from build123d import *

# Parameters (mm, degrees)
BOSS_EXTRUDE1_DEPTH            = 9.6
SKETCH2_W                      = 21
SKETCH2_H                      = 15
BOSS_EXTRUDE2_DEPTH            = 2
SKETCH3_W                      = 18.8
SKETCH3_H                      = 13
BOSS_EXTRUDE3_DEPTH            = 13.5
SKETCH4_W                      = 1
SKETCH4_H                      = 4.8
BOSS_EXTRUDE4_DEPTH            = 8
SKETCH5_W                      = 1
SKETCH5_H                      = 4.8
BOSS_EXTRUDE5_DEPTH            = 8
SKETCH6_W                      = 1
SKETCH6_H                      = 4.8
BOSS_EXTRUDE6_DEPTH            = 8
F_1_6_1_6_DIAMETER_HOLE1_D     = 1.6
F_1_6_1_6_DIAMETER_HOLE1_DEPTH = 1
F_1_6_1_6_DIAMETER_HOLE2_D     = 1.6
F_1_6_1_6_DIAMETER_HOLE2_DEPTH = 1
F_1_6_1_6_DIAMETER_HOLE3_D     = 1.6
F_1_6_1_6_DIAMETER_HOLE3_DEPTH = 11
CHAMFER1_SIZE                  = 0.25
CHAMFER2_SIZE                  = 0.5


with BuildPart() as part:
    # Sketch1 → Boss-Extrude1 (new body)
    with BuildSketch(Plane(origin=(0, 0, -4.8), x_dir=(-1, 0, 0), z_dir=(0, 0, -1))):
        with BuildLine():
            Line((-7.639445546, 15.5), (6.803913489, 15.5))
            ThreePointArc((6.803913489, 15.5), (1.329165769, 16.958613053), (-3.894073755, 19.15364916))
            ThreePointArc((-3.894073755, 19.15364916), (-6.290531384, 17.863745283), (-7.639445546, 15.5))
        make_face()
    extrude(amount=-BOSS_EXTRUDE1_DEPTH)

    # Sketch2 → Boss-Extrude2 (add)
    with BuildSketch(Plane(origin=(0, 15.5, 0), x_dir=(1, 0, 0), z_dir=(0, 1, 0))):
        Rectangle(SKETCH2_W, SKETCH2_H)
    extrude(amount=-BOSS_EXTRUDE2_DEPTH)

    # Sketch3 → Boss-Extrude3 (add)
    with BuildSketch(Plane.XZ.offset(-13.5)):
        Rectangle(SKETCH3_W, SKETCH3_H)
    extrude(amount=BOSS_EXTRUDE3_DEPTH)

    # Sketch4 → Boss-Extrude4 (add)
    with BuildSketch(Plane.XZ):
        Rectangle(SKETCH4_W, SKETCH4_H)
    extrude(amount=BOSS_EXTRUDE4_DEPTH)

    # Sketch5 → Boss-Extrude5 (add)
    with BuildSketch(Plane.XZ):
        with Locations((7.1, 0)):
            Rectangle(SKETCH5_W, SKETCH5_H)
    extrude(amount=BOSS_EXTRUDE5_DEPTH)

    # Sketch6 → Boss-Extrude6 (add)
    with BuildSketch(Plane.XZ):
        with Locations((-7.1, 0)):
            Rectangle(SKETCH6_W, SKETCH6_H)
    extrude(amount=BOSS_EXTRUDE6_DEPTH)

    # Ø1.6 (1.6) Diameter Hole1
    with Locations(Plane.ZY.offset(7.6)):
        with Locations((0, -4.5)):
            Hole(F_1_6_1_6_DIAMETER_HOLE1_D / 2, depth=F_1_6_1_6_DIAMETER_HOLE1_DEPTH)

    # Ø1.6 (1.6) Diameter Hole2
    with Locations(Plane(origin=(7.6, 0, 0), x_dir=(0, 0, -1), z_dir=(1, 0, 0))):
        with Locations((0, -4.5)):
            Hole(F_1_6_1_6_DIAMETER_HOLE2_D / 2, depth=F_1_6_1_6_DIAMETER_HOLE2_DEPTH)

    # Ø1.6 (1.6) Diameter Hole3
    with Locations(Plane.ZY.offset(0.5)):
        with Locations((0, -4.5)):
            Hole(F_1_6_1_6_DIAMETER_HOLE3_D / 2, depth=F_1_6_1_6_DIAMETER_HOLE3_DEPTH)

    # Chamfer1
    chamfer1_edges = [part.edges().sort_by_distance(p)[0] for p in [
        (-0.5, -8, 0),
        (0.5, -8, 0),
        (6.6, -8, 0),
        (7.6, -8, 0),
    ]]
    chamfer(chamfer1_edges, length=CHAMFER1_SIZE)

    # Chamfer2
    chamfer2_edges = [part.edges().sort_by_distance(p)[0] for p in [
        (7.1, -8, 2.4),
        (-7.1, -8, -2.4),
        (7.1, -8, -2.4),
        (0, -8, -2.4),
        (-7.1, -8, 2.4),
        (0, -8, 2.4),
    ]]
    chamfer(chamfer2_edges, length=CHAMFER2_SIZE)


solid = part.part
Input: part model. Units: mm. Frame: model coordinates. A direction names the side the tool comes from. Coordinates: 2 decimals unless noted, no trailing zeros. Loops run counter-clockwise (first coordinate to the right, second up) from the corner with the lowest first, then second, coordinate; pieces in that order, holes last. Notation, with made-up numbers: (32.5, -20) - (73.5, -20) arc R32 cw to (73.5, 12) - close; hole circle Ø5 at (62.25, -16.5). An arc over 180 degrees is marked (long way). Answer in a Markdown table with one row per item. Add a question column.
Item 1: Mould query, pull axis Z, two halves, no side actions, for faces 1 (the cylindrical face through (-1.404, 16.933, -0.067)), 2 (the flat face through (0, 7, 6.5)), 3 (the cylindrical face through (-7.09, -5.28, 0.17)). Classes: released by +Z, released by -Z, zero draft, split by the parting line, or undercut.
Item 2: Section query A-A on y = -4.5. Return the cut outline in (x, z).
Item 3: Section query B-B on z = -3. Return the cut outline in (x, y).
Item 4: Contact query for flat-ended pins moving along their axis: P1, Ø4, axis at x = 2, y = -2.5, coming from the +Z side; P2, Ø1.4, axis at y = -3.5, z = -1, coming from the -X side; P3, Ø4, axis at x = 2, z = -5.5, coming from the +Y side; P4, Ø1.4, axis at y = -4.5, z = 0, coming from the +X side. Output: stop coordinate, or through.
Item 5: Section query D-D on z = 0. State how many separate pieces and enclosed holes the cut face has, then the cut area to 3 significant figures.
Item 6: Section query C-C on x = -5. Return the cut outline in (y, z), then the cut area to 3 significant figures.
Item 7: Line query: line 1 along X through (y, z) = (-6.75, 0); line 2 along Y through (x, z) = (-7.25, 0); line 3 along Z through (x, y) = (7, -4.5). Output: solid intervals per line, ascending. Write a range as [from, to].
Item 8: Access query for faces 4 (the flat face through (-7.6, -3, 0)), 5 (the flat face through (-6.6, -3, 0)), 6 (the flat face through (-7, -4, 2.4)), 7 (the flat face through (2, 17, -4.8)). Directions: +Z, -Z, +X, -X, +Y, -Y. A direction counts if a zero-diameter tool reaches every point of the face in a straight line with its end or side. Return the directions, or none.
Recorded:
| question | item | result |
|---|---|---|
| 1 | face 1 | zero draft |
| 1 | face 2 | released by +Z |
| 1 | face 3 | undercut |
| 2 | outline | (-7.6, -2.4) - (-6.6, -2.4) - (-6.6, -0.8) - (-7.6, -0.8) - close; (-7.6, 0.8) - (-6.6, 0.8) - (-6.6, 2.4) - (-7.6, 2.4) - close; (-0.5, -2.4) - (0.5, -2.4) - (0.5, -0.8) - (-0.5, -0.8) - close; (-0.5, 0.8) - (0.5, 0.8) - (0.5, 2.4) - (-0.5, 2.4) - close; (6.6, -2.4) - (7.6, -2.4) - (7.6, -0.8) - (6.6, -0.8) - close; (6.6, 0.8) - (7.6, 0.8) - (7.6, 2.4) - (6.6, 2.4) - close |
| 3 | outline | (-10.5, 13.5) - (-9.4, 13.5) - (-9.4, 0) - (9.4, 0) - (9.4, 13.5) - (10.5, 13.5) - (10.5, 15.5) - (7.64, 15.5) arc R4.94 ccw to (3.89, 19.15) arc R41.25 cw to (-6.8, 15.5) - (-10.5, 15.5) - close |
| 4 | P1 | z = 2.4 |
| 4 | P2 | x = -7.6 |
| 4 | P3 | y = 19.14 |
| 4 | P4 | through |
| 5 | separate pieces | 4 |
| 5 | enclosed holes | 0 |
| 5 | area | 341 mm^2 |
| 6 | outline | (0, -6.5) - (13.5, -6.5) - (13.5, -7.5) - (15.5, -7.5) - (15.5, -4.8) - (15.89, -4.8) - (15.89, 4.8) - (15.5, 4.8) - (15.5, 7.5) - (13.5, 7.5) - (13.5, 6.5) - (0, 6.5) - close |
| 6 | area | 209 mm^2 |
| 7 | line 1 | [-7.6, -6.6], [-0.5, 0.5], [6.6, 7.6] |
| 7 | line 2 | [-8, -5.3], [-3.7, 15.5] |
| 7 | line 3 | [-2.4, -0.8], [0.8, 2.4] |
| 8 | face 4 | +Z, -Z, -X, -Y |
| 8 | face 5 | +Z, -Z, -Y |
| 8 | face 6 | +Z, +X, -X, -Y |
| 8 | face 7 | -Z, +X, -X, +Y |
